Geometry check sheet. Reference: the model listing, model coordinates, mm. A direction names the side the tool comes from. Round coordinates to 2 decimals unless told otherwise and drop trailing zeros. Loops run counter-clockwise (first coordinate to the right, second up) from the corner with the lowest first, then second, coordinate; pieces in that order, holes last. Notation, with made-up numbers: (6.5, 59.5) - (38.5, 59.5) arc R17 cw to (38.5, 64.5) - close; hole circle Ø1 at (-21.5, -21.5). An arc over 180 degrees is marked (long way). Answer in a Markdown table with one row per item. Add a question column.
```python
from build123d import *

# Parameters (mm, degrees)
F0_R      = 51.7
F0_R_2    = 40
F0_R_3    = 22.5
F1_DEPTH  = 57
F2_DEPTH  = 10
F3_DEPTH  = 16
F4_R      = 50
F4_R_2    = 45
F5_DEPTH  = 37
F6_DEPTH  = 41
F4_R_3    = 100
F4_R_4    = 92
F4_R_5    = 60
F4_R_6    = 51.7
F7_DEPTH  = 5
F8_DEPTH  = 3
F9_R      = 116.2259856664
F10_DEPTH = 10


# Not quite as in the source:
# - a feature names something its author has since deleted; it is built from what else it names


with BuildPart() as f1:
    # F0 (on Front) → F1 (new body)
    with BuildSketch(Plane.XZ):
        Circle(F0_R)
        Circle(F0_R_2, mode=Mode.SUBTRACT)
        Circle(F0_R_2)
        Circle(F0_R_3, mode=Mode.SUBTRACT)
        Circle(F0_R_3)
    extrude(amount=-F1_DEPTH)

    # F0 (on Front) → F2 (cut)
    with BuildSketch(Plane.XZ):
        Circle(F0_R_2)
        Circle(F0_R_3, mode=Mode.SUBTRACT)
    extrude(amount=-F2_DEPTH, mode=Mode.SUBTRACT)

    # F0 (on Front) → F3 (cut)
    with BuildSketch(Plane.XZ):
        Circle(F0_R_3)
    extrude(amount=-F3_DEPTH, mode=Mode.SUBTRACT)

    # F4 (on face) → F5 (cut)
    with BuildSketch(Plane(origin=(0, 57, 0), x_dir=(-1, 0, 0), z_dir=(0, 1, 0))):
        Circle(F4_R)
        Circle(F4_R_2, mode=Mode.SUBTRACT)
    extrude(amount=-F5_DEPTH, mode=Mode.SUBTRACT)

    # F4 (on face) → F6 (cut)
    with BuildSketch(Plane(origin=(0, 57, 0), x_dir=(-1, 0, 0), z_dir=(0, 1, 0))):
        Circle(F4_R_2)
    extrude(amount=-F6_DEPTH, mode=Mode.SUBTRACT)

    # F4 (on face) → F7 (join)
    with BuildSketch(Plane(origin=(0, 57, 0), x_dir=(-1, 0, 0), z_dir=(0, 1, 0))):
        Circle(F4_R_3)
        Circle(F4_R_4, mode=Mode.SUBTRACT)
        Circle(F4_R_4)
        Circle(F4_R_5, mode=Mode.SUBTRACT)
        Circle(F4_R_5)
        Circle(F4_R_6, mode=Mode.SUBTRACT)
    extrude(amount=-F7_DEPTH)

    # F4 (on face) → F8 (cut)
    with BuildSketch(Plane(origin=(0, 57, 0), x_dir=(-1, 0, 0), z_dir=(0, 1, 0))):
        Circle(F4_R_4)
        Circle(F4_R_5, mode=Mode.SUBTRACT)
    extrude(amount=-F8_DEPTH, mode=Mode.SUBTRACT)

    # F9 (on face) → F10 (join)
    with BuildSketch(Plane.XZ.offset(-52)):
        with Locations((4.3108635582, 0)):
            Circle(F9_R)
    extrude(amount=F10_DEPTH)


solid = f1.part
```
Q1. Cross-section at A-A, the plane z = 79. Enter the section's corners in (x, y).
Q2. Release check for a two-part mould opening along X. For faces 6 (the flat face through (17, 10, -17)), 7 (the cylindrical face through (-47.69, 31.15, 15.02)), 8 (the cylindrical face through (-11.21, 20.71, -50.47)), 9 (the flat face through (23, 57, 45)) record: +X half, -X half, draft (parallel to the pull), parting line (faces both ways), or undercut.
Q3. Scan lines: line 1 (Z direction, x = 0, y = 54.9); line 2 (Y direction, x = -47, z = -5.5); line 3 (Y direction, x = -71.5, z = 44). Record each from-to range of solid material in increasing order. Write a range as from..to.
Q4. Cross-section at D-D, the plane z = 55. Enter the section's corners in (x, y), plus the area to 3 significant figures.
Q5. Set-up check for faces 1 (the flat face through (41, 20, 19)), 2 (the flat face through (-60, 54, -19)), 3 (the flat face through (27, 0, -30)), 4 (the cylindrical face through (-20.885, 47.07, -113.462)), 5 (the flat face through (54, 42, 2)): record each of +Z, -Z, +X, -X, +Y, -Y from which the full face is reachable in a straight line by a thin tool's end or side.
Q6. Cross-section at B-B, the plane y = 47. Enter the section's corners in (x, z), plus the area to 3 significant figures.
Q7. Cross-section at C-C, the plane x = -55.5. Enter the section's corners in (y, z), plus the area to 3 significant figures.
Q8. Depth check by flat-ended pin: P1, Ø1.5, axis at x = 58, y = 49.5, coming from the +Z side; P2, Ø8, axis at x = 12.5, y = 36.5, coming from the +Z side; P3, Ø10, axis at x = -59, y = 43.5, coming from the -Z side. Enter the tip coordinate at first touch or a pass-through.
Check sheet entries:
| question | item | result |
|---|---|---|
| 1 | outline | (-80.94, 42) - (89.56, 42) - (89.56, 52) - (61.31, 52) - (61.31, 57) - (47.15, 57) - (47.15, 54) - (-47.15, 54) - (-47.15, 57) - (-61.31, 57) - (-61.31, 52) - (-80.94, 52) - close |
| 2 | face 6 | undercut |
| 2 | face 7 | undercut |
| 2 | face 8 | parting line |
| 2 | face 9 | draft |
| 3 | line 1 | -100..-92, -60..-50, 50..60, 92..100 |
| 3 | line 2 | 0..20, 42..52 |
| 3 | line 3 | 42..54 |
| 4 | outline | (-98.08, 42) - (106.7, 42) - (106.7, 52) - (83.52, 52) - (83.52, 57) - (73.75, 57) - (73.75, 54) - (23.98, 54) - (23.98, 57) - (-23.98, 57) - (-23.98, 54) - (-73.75, 54) - (-73.75, 57) - (-83.52, 57) - (-83.52, 52) - (-98.08, 52) - close |
| 4 | area | 2,580 mm² |
| 5 | face 1 | none |
| 5 | face 2 | +Y |
| 5 | face 3 | +Z, -Z, +X, -X, -Y |
| 5 | face 4 | +Y, -Y |
| 5 | face 5 | -Y |
| 6 | outline | circle Ø232.45 at (4.31, 0) |
| 6 | area | 42,400 mm² |
| 7 | outline | (42, -99.66) - (52, -99.66) - (52, -83.19) - (57, -83.19) - (57, -73.37) - (54, -73.37) - (54, -22.8) - (57, -22.8) - (57, 22.8) - (54, 22.8) - (54, 73.37) - (57, 73.37) - (57, 83.19) - (52, 83.19) - (52, 99.66) - (42, 99.66) - close |
| 7 | area | 2,520 mm² |
| 8 | P1 | z = 103.47 |
| 8 | P2 | z = 51 |
| 8 | P3 | z = -100.54 |
